Check sheet for the modelled part. Datum: model origin and axes. Units: mm. Face numbers are marked on the shaded views. A direction names the side the tool comes from. Round coordinates to 2 decimals unless told otherwise and drop trailing zeros. Write each loop counter-clockwise with the first axis right and the second up, starting at its lowest first coordinate (ties: lowest second). Pieces come first, ordered by that corner, then holes. Notation, with made-up numbers: M 39.5,-7.75 L 68.5,-7.75 A7 ccw 68.5,-3.75 Z; hole C 36,24 d3. An arc over 180 degrees is marked long. Answer in a Markdown table with one row per item.
```python
from build123d import *

# Parameters (mm, degrees)
F0_W     = 71.5
F0_H     = 43.5
F1_DEPTH = 29
F2_W     = 50
F2_H     = 43.5
F3_DEPTH = 14.5
F4_W     = 21
F4_H     = 13.5
F5_DEPTH = 14.501


with BuildPart() as f1:
    # F0 (on Top) → F1 (new body)
    with BuildSketch(Plane.XY):
        with Locations((35.75, 21.75)):
            Rectangle(F0_W, F0_H)
    extrude(amount=F1_DEPTH)

    # F2 (on face) → F3 (cut)
    with BuildSketch(Plane.XY.offset(29)):
        with Locations((46.5, 21.75)):
            Rectangle(F2_W, F2_H)
    extrude(amount=-F3_DEPTH, mode=Mode.SUBTRACT)

    # F4 (on face) → F5 (cut, through all)
    with BuildSketch(Plane.XY.offset(14.5)):
        with Locations((61, 6.75)):
            Rectangle(F4_W, F4_H)
    extrude(amount=-F5_DEPTH, mode=Mode.SUBTRACT)


solid = f1.part
```
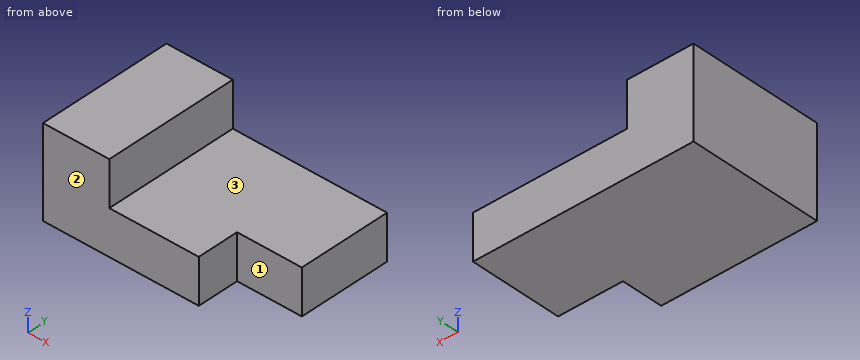
1. Scan lines: L1, parallel to X at y = 4, z = 15.5; L2, parallel to Z at x = 33, y = 27; L3, parallel to X at y = 11.5, z = 12.5. Record each from-to range of solid material in increasing order.
Found:
| item | result |
|---|---|
| L1 | x = 0 to 21.5 |
| L2 | z = 0 to 14.5 |
| L3 | x = 0 to 50.5 |
2. Go/stop test with flat-tipped pins: pin 1 (7 mm diameter, centred on y = 15, z = 20, fed in from +X); pin 2 (4 mm diameter, centred on y = 9, z = 9, fed in from +X); pin 3 (4.5 mm diameter, centred on x = 64.5, z = 7.5, fed in from -Y); pin 4 (10 mm diameter, centred on x = 41, z = 22.5, fed in from -Y). Record where each tip stops, or that it passes through.
Found:
| item | result |
|---|---|
| pin 1 | stops at x = 21.5 |
| pin 2 | stops at x = 50.5 |
| pin 3 | stops at y = 13.5 |
| pin 4 | passes through |
3. Section check D-D, the plane z = 15.5. Record the cut outline in (x, y).
Found:
| item | result |
|---|---|
| outline | M 0,0 L 21.5,0 L 21.5,43.5 L 0,43.5 Z |
4. Access from +Z, -Z, +X, -X, +Y, -Y to the whole of each face (thin tool, end or side, straight path). Record for the marked faces 1, 2 and 3.
Found:
| item | result |
|---|---|
| face 1 | +Z, -Z, +X, -Y |
| face 2 | +Z, -Z, +X, -X, -Y |
| face 3 | +Z, +X, +Y, -Y |
5. Section check A-A, the plane y = 30.5. Record the cut outline in (x, z), and give its area (3 significant figures).
Found:
| item | result |
|---|---|
| outline | M 0,0 L 71.5,0 L 71.5,14.5 L 21.5,14.5 L 21.5,29 L 0,29 Z |
| area | 1,350 mm2 |
6. Section check C-C, the plane x = 46.5. Record the cut outline in (y, z), and give its area (3 significant figures).
Found:
| item | result |
|---|---|
| outline | M 0,0 L 43.5,0 L 43.5,14.5 L 0,14.5 Z |
| area | 631 mm2 |
7. Section check B-B, the plane z = 8. Record the cut outline in (x, y), and give its area (3 significant figures).
Found:
| item | result |
|---|---|
| outline | M 0,0 L 50.5,0 L 50.5,13.5 L 71.5,13.5 L 71.5,43.5 L 0,43.5 Z |
| area | 2,830 mm2 |
